Here's the drawing with two shaded views (mm, measured from the low corner). I have some questions. Coordinates: 2 decimals unless noted, no trailing zeros. Loops run counter-clockwise (first coordinate to the right, second up) from the corner with the lowest first, then second, coordinate; pieces in that order, holes last. Notation, with made-up numbers: (-36.75, -39) -> (-11.75, -39) arc R9 ccw to (-11.75, -35) -> close; hole circle Ø5 at (-35, -13). An arc over 180 degrees is marked (long way). Answer as a JSON object with one key per item and string values. Group by question number.
1) I need wall thicknesses on probe 1 along X at (y, z) = (70.5, 243.5); probe 2 along Z at (x, y) = (803, 124) (1 decimal); probe 3 along Z at (x, y) = (715, 80.5) (3 decimals). Which ranges of each line are inside material? Lowest first, please. Write a range as [from, to].
2) I'm going to push flat-ended pins straight in: pin 1 (2 mm diameter, centred on y = 78.5, z = 105.5, fed in from -X); pin 2 (1 mm diameter, centred on y = 74, z = 273.5, fed in from +X); pin 3 (6 mm diameter, centred on y = 107.5, z = 276.5, fed in from +X). Where does each tip first touch, or does it pass through?
3) I want a section at B-B (x = 419.5). Write out the boundary of the cut face in (y, z).
4) I want a section at A-A (y = 86). Write out the boundary of the cut face in (x, z).
5) I want a section at C-C (y = 124). Write out the boundary of the cut face in (x, z), then the cut area to 3 significant figures.
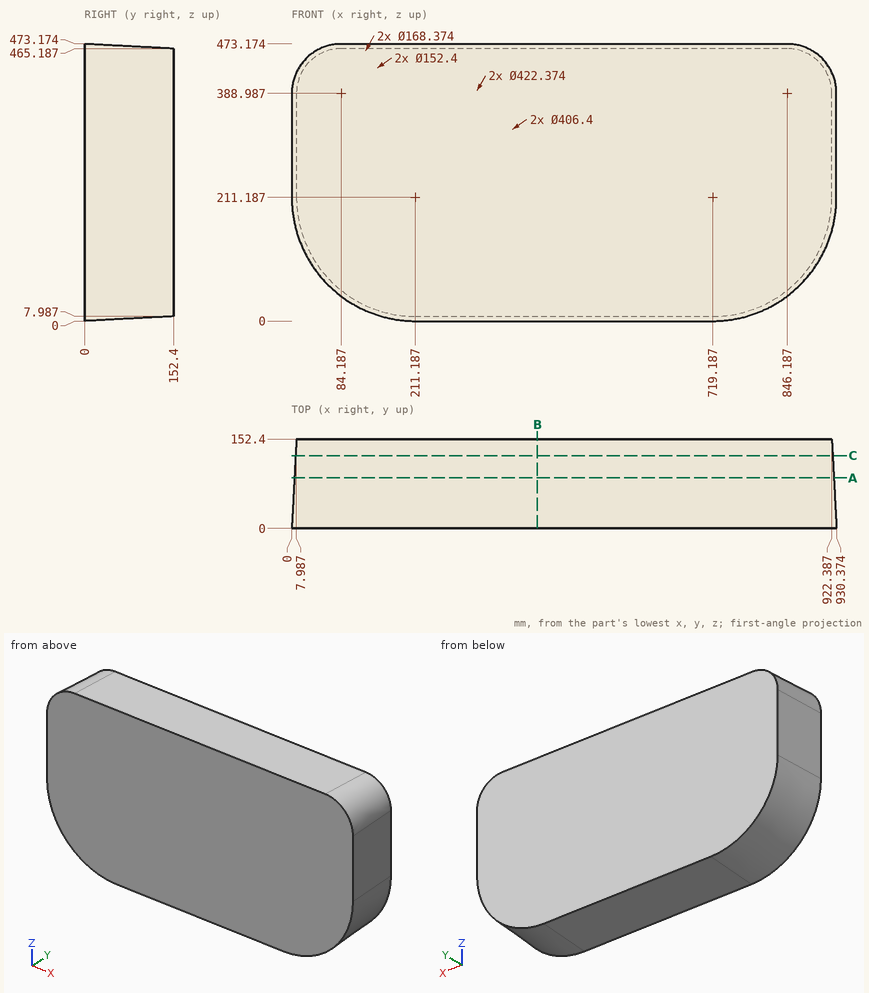
Determined:
{
 "1": {"probe 1": "[3.69, 926.68]", "probe 2": "[24.4, 466.7]", "probe 3": "[4.219, 468.955]"},
 "2": {"pin 1": "x = 32.52", "pin 2": "x = 926.52", "pin 3": "x = 924.9"},
 "3": {"outline": "(0, 0) -> (152.4, 7.99) -> (152.4, 465.19) -> (0, 473.17) -> close"},
 "4": {"outline": "(4.51, 211.19) arc R206.68 ccw to (211.19, 4.51) -> (719.19, 4.51) arc R206.68 ccw to (925.87, 211.19) -> (925.87, 388.99) arc R79.68 ccw to (846.19, 468.67) -> (84.19, 468.67) arc R79.68 ccw to (4.51, 388.99) -> close"},
 "5": {"outline": "(6.5, 211.19) arc R204.69 ccw to (211.19, 6.5) -> (719.19, 6.5) arc R204.69 ccw to (923.88, 211.19) -> (923.88, 388.99) arc R77.69 ccw to (846.19, 466.68) -> (84.19, 466.68) arc R77.69 ccw to (6.5, 388.99) -> close", "area": "402,000 mm^2"}
}
